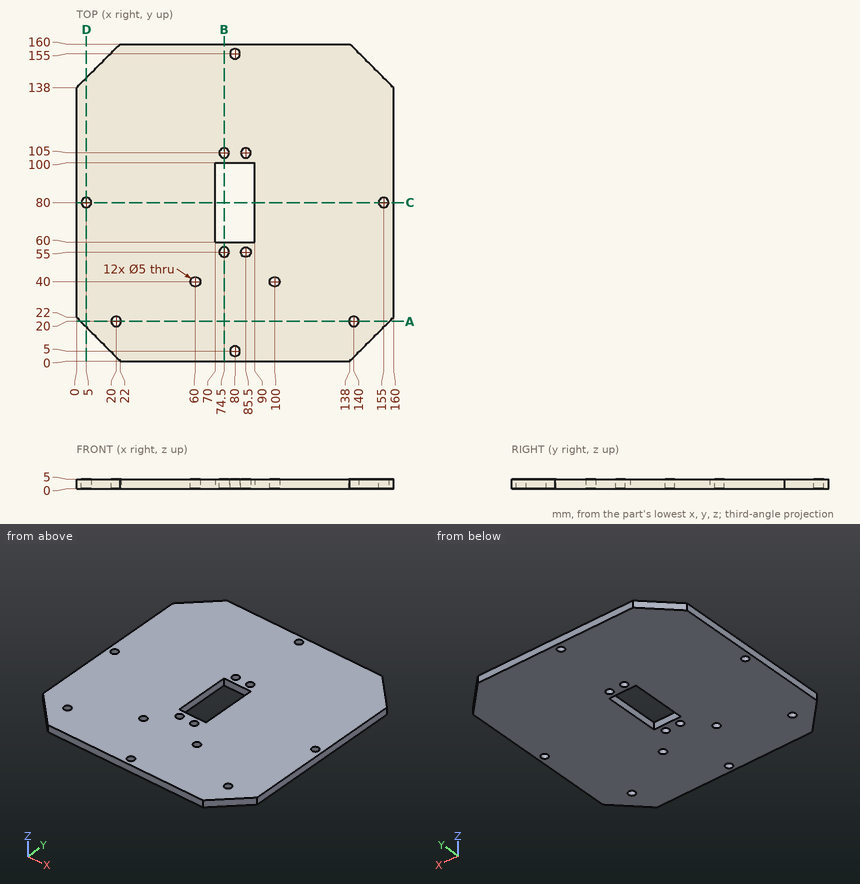
Job drawing, mm, ordinate dimensions from the low corner. One solid piece. Round coordinates to 2 decimals unless told otherwise and drop trailing zeros. Order: outer loops, then holes, each group sorted by start corner. A loop starts at its lowest first (then second) coordinate and runs counter-clockwise, first axis right, second up. Notation, with made-up numbers: M 65,-32.5 L 83,-32.5 A13 ccw 83,-19.5 Z; hole C 37,11 d11. An arc over 180 degrees is marked long. Write each question's results on one line, items separated by ' | '. Start each with the question number.
(1) Drop flat-ended pins along their axis: pin 1 (6 mm diameter, centred on x = 74.5, y = 105, fed in from +Z); pin 2 (3 mm diameter, centred on y = 19, z = 3.5, fed in from +X); pin 3 (3 mm diameter, centred on x = 20, y = 20, fed in from +Z). Give the stop position or say it passes through.
(2) Saw through at D-D, the plane x = 5. Give the cut face in (y, z).
(3) Saw through at C-C, the plane y = 80. Give the cut face in (x, z), then the cut area to 3 significant figures.
(4) Saw through at A-A, the plane y = 20. Give the cut face in (x, z).
(5) Probe probe 1 along X at (y, z) = (105, 1.85); probe 2 along X at (y, z) = (40, 1.95); probe 3 along Y at (x, z) = (74.5, 1.2). List the from-to ranges inside material, lowest first. Write a range as from..to.
(6) Saw through at B-B, the plane x = 74.5. Give the cut face in (y, z), then the cut area to 3 significant figures.
Established:
1) pin 1: stops at z = 5 | pin 2: stops at x = 158.5 | pin 3: passes through
2) outline: M 17,0 L 77.5,0 L 77.5,5 L 17,5 Z; M 82.5,0 L 143,0 L 143,5 L 82.5,5 Z
3) outline: M 0,0 L 2.5,0 L 2.5,5 L 0,5 Z; M 7.5,0 L 70,0 L 70,5 L 7.5,5 Z; M 90,0 L 152.5,0 L 152.5,5 L 90,5 Z; M 157.5,0 L 160,0 L 160,5 L 157.5,5 Z | area: 650 mm^2
4) outline: M 2,0 L 17.5,0 L 17.5,5 L 2,5 Z; M 22.5,0 L 137.5,0 L 137.5,5 L 22.5,5 Z; M 142.5,0 L 158,0 L 158,5 L 142.5,5 Z
5) probe 1: x = 0..72, 77..83, 88..160 | probe 2: x = 0..57.5, 62.5..97.5, 102.5..160 | probe 3: y = 0..52.5, 57.5..60, 100..102.5, 107.5..160
6) outline: M 0,0 L 52.5,0 L 52.5,5 L 0,5 Z; M 57.5,0 L 60,0 L 60,5 L 57.5,5 Z; M 100,0 L 102.5,0 L 102.5,5 L 100,5 Z; M 107.5,0 L 160,0 L 160,5 L 107.5,5 Z | area: 550 mm^2
